```python
from build123d import *

# Parameters (mm, degrees)
SKETCH_1_W          = 19
SKETCH_1_H          = 19
SKETCH_1_R          = 1
EXTRUDE_1_DEPTH     = 6
FILLET_1_R          = 1
SKETCH_2_R          = 1
CUT_EXTRUDE_1_DEPTH = 28.531799796
CUT_EXTRUDE_2_DEPTH = 3


with BuildPart() as part:
    # Эскиз1 → Бобышка-Вытянуть1 (new body)
    with BuildSketch(Plane(origin=(0, 0, 0), x_dir=(1, 0, 0), z_dir=(0, 1, 0))):
        with Locations((9.5, 9.5)):
            Rectangle(SKETCH_1_W, SKETCH_1_H)
        with Locations(Location((2, 17, 0), (0, 0, 270))):
            Circle(SKETCH_1_R, mode=Mode.SUBTRACT)
        with Locations(Location((17, 17, 0), (0, 0, 270))):
            Circle(SKETCH_1_R, mode=Mode.SUBTRACT)
        with Locations(Location((17, 2, 0), (0, 0, 270))):
            Circle(SKETCH_1_R, mode=Mode.SUBTRACT)
        with Locations(Location((2, 2, 0), (0, 0, 270))):
            Circle(SKETCH_1_R, mode=Mode.SUBTRACT)
    extrude(amount=EXTRUDE_1_DEPTH)

    # Скругление1
    fillet_1_edges = [part.edges().sort_by_distance(p)[0] for p in [
        (0, 3, -19),
        (19, 3, -19),
        (19, 3, 0),
        (0, 3, 0),
    ]]
    fillet(fillet_1_edges, radius=FILLET_1_R)

    # Эскиз2 → Вырез-Вытянуть1 (cut, through all)
    with BuildSketch(Plane(origin=(0, 6, 0), x_dir=(1, 0, 0), z_dir=(0, 1, 0))):
        with Locations(Location((9.5, 16.5, 0), (0, 0, 270))):
            Circle(SKETCH_2_R)
        with Locations(Location((16.5, 9.5, 0), (0, 0, 270))):
            Circle(SKETCH_2_R)
        with Locations(Location((9.5, 2.5, 0), (0, 0, 270))):
            Circle(SKETCH_2_R)
        with Locations(Location((2.5, 9.5, 0), (0, 0, 270))):
            Circle(SKETCH_2_R)
    extrude(amount=-CUT_EXTRUDE_1_DEPTH, mode=Mode.SUBTRACT)

    # Эскиз3 → Вырез-Вытянуть2 (cut)
    with BuildSketch(Plane(origin=(0, 6, 0), x_dir=(1, 0, 0), z_dir=(0, 1, 0))):
        with BuildLine():
            Line((6, 16.5), (6, 21.9359466))
            Line((6, 21.9359466), (13, 21.9359466))
            Line((13, 21.9359466), (13, 16.5))
            ThreePointArc((13, 16.5), (9.5, 13), (6, 16.5))
        make_face()
        with BuildLine():
            Line((13, 2.5), (13, -5.102937302))
            Line((13, -5.102937302), (6, -4.799159297))
            Line((6, -4.799159297), (6, 2.5))
            ThreePointArc((6, 2.5), (9.5, 6), (13, 2.5))
        make_face()
        with BuildLine():
            Line((2.5, 6), (-3.698936954, 6))
            Line((-3.698936954, 6), (-3.698936954, 13))
            Line((-3.698936954, 13), (2.5, 13))
            ThreePointArc((2.5, 13), (6, 9.5), (2.5, 6))
        make_face()
        with BuildLine():
            Line((22.836899795, 13), (22.836899795, 6))
            Line((22.836899795, 6), (16.5, 6))
            ThreePointArc((16.5, 6), (13, 9.5), (16.5, 13))
            Line((16.5, 13), (22.836899795, 13))
        make_face()
    extrude(amount=-CUT_EXTRUDE_2_DEPTH, mode=Mode.SUBTRACT)


solid = part.part
```
Geometry check sheet. Reference: the model listing, model coordinates, mm. A direction names the side the tool comes from. Round coordinates to 2 decimals unless told otherwise and drop trailing zeros. Loops run counter-clockwise (first coordinate to the right, second up) from the corner with the lowest first, then second, coordinate; pieces in that order, holes last. Notation, with made-up numbers: (-18, 74.25) - (38, 74.25) arc R15 cw to (38, 95.25) - close; hole circle Ø11 at (-28.5, 28). An arc over 180 degrees is marked (long way). Write item = value, one per line. Start each with the question number.
1. Section check A-A on z = -9.5. Enter the section's corners in (x, y), then the cut area to 3 significant figures.
2. Depth check by flat-ended pin: pin 1 (3 mm diameter, centred on x = 8.5, z = -15, fed in from +Y); pin 2 (1.8 mm diameter, centred on x = 9.5, z = -16.5, fed in from +Y); pin 3 (0.8 mm diameter, centred on y = 4, z = -18.5, fed in from +X) (3 decimals). Enter the tip coordinate at first touch or a pass-through.
3. Section check D-D on y = 4.45. Enter the section's corners in (x, z), then the cut area to 3 significant figures.
4. Set-up check for faces 4 (the face through (18, 5, -6)), 5 (the face through (13, 5, -1)), 6 (the face through (9.6, 4.5, -13)), 7 (the face through (4, 3, -10)): record each of +Z, -Z, +X, -X, +Y, -Y from which the full face is reachable in a straight line by a thin tool's end or side.
5. Section check C-C on x = 2.25. Enter the section's corners in (y, z).
6. Thickness scan on line 1 (X direction, y = 4.8, z = -17); line 2 (Z direction, x = 2.25, y = 1.5); line 3 (X direction, y = 1.35, z = -2.5). Record the ranges inside material, lowest first.
7. Mould release check, pull along Z, two halves, no side actions. Record for faces 1 (the face through (10.49, 1.52, -2.63)), 2 (the face through (9, 0, -10)), 3 (the face through (9, 2, 0)): released by +Z, released by -Z, zero draft, split by the parting line, or undercut.
8. Section check B-B on y = 0.5. Give the number of separate pieces and of enclosed holes in the cut face, then the cut area to 3 significant figures.
Working result:
q1.outline = (0, 0) - (1.5, 0) - (1.5, 3) - (0, 3) - close; (3.5, 0) - (15.5, 0) - (15.5, 3) - (13, 3) - (13, 6) - (6, 6) - (6, 3) - (3.5, 3) - close; (17.5, 0) - (19, 0) - (19, 3) - (17.5, 3) - close
q1.area = 66.0 mm^2
q2.pin_1 = 3
q2.pin_2 = through
q2.pin_3 = 18.995
q3.outline = (0, -18) arc R1 ccw to (1, -19) - (6, -19) - (6, -16.5) arc R3.5 cw to (13, -16.5) - (13, -19) - (18, -19) arc R1 ccw to (19, -18) - (19, -13) - (16.5, -13) arc R3.5 cw to (16.5, -6) - (19, -6) - (19, -1) arc R1 ccw to (18, 0) - (13, 0) - (13, -2.5) arc R3.5 cw to (6, -2.5) - (6, 0) - (1, 0) arc R1 ccw to (0, -1) - (0, -6) - (2.5, -6) arc R3.5 cw to (2.5, -13) - (0, -13) - close; hole circle Ø2 at (2, -17); hole circle Ø2 at (2, -2); hole circle Ø2 at (17, -17); hole circle Ø2 at (17, -2)
q3.area = 201 mm^2
q4.face_4 = +X, +Y
q4.face_5 = +Z, +Y
q4.face_6 = -Z, +Y
q4.face_7 = -X, +Y
q5.outline = (0, -19) - (6, -19) - (6, -17.97) - (0, -17.97) - close; (0, -16.03) - (6, -16.03) - (6, -13) - (3, -13) - (3, -10.47) - (0, -10.47) - close; (0, -8.53) - (3, -8.53) - (3, -6) - (6, -6) - (6, -2.97) - (0, -2.97) - close; (0, -1.03) - (6, -1.03) - (6, 0) - (0, 0) - close
q6.line_1 = 0 to 1, 3 to 6, 13 to 16, 18 to 19
q6.line_2 = -19 to -17.97, -16.03 to -10.47, -8.53 to -2.97, -1.03 to 0
q6.line_3 = 0 to 1.13, 2.87 to 8.5, 10.5 to 16.13, 17.87 to 19
q7.face_1 = undercut
q7.face_2 = zero draft
q7.face_3 = released by +Z
q8.separate_pieces = 1
q8.enclosed_holes = 8
q8.area = 335 mm^2
